The drawing under review shows one solid part. Ordinate dimensions are in mm from its lowest x, y, z. A direction names the side the tool comes from. Give positions to 0.01 mm unless a question says otherwise; leave off trailing zeros. Write each loop counter-clockwise with the first axis right and the second up, starting at its lowest first coordinate (ties: lowest second). Pieces come first, ordered by that corner, then holes. Notation, with made-up numbers: (85.5, 4.5) -> (104.5, 4.5) arc R23 cw to (104.5, 29.5) -> close; hole circle Ø4 at (-1, -13.75). An arc over 180 degrees is marked (long way). Write item = value, one per line.
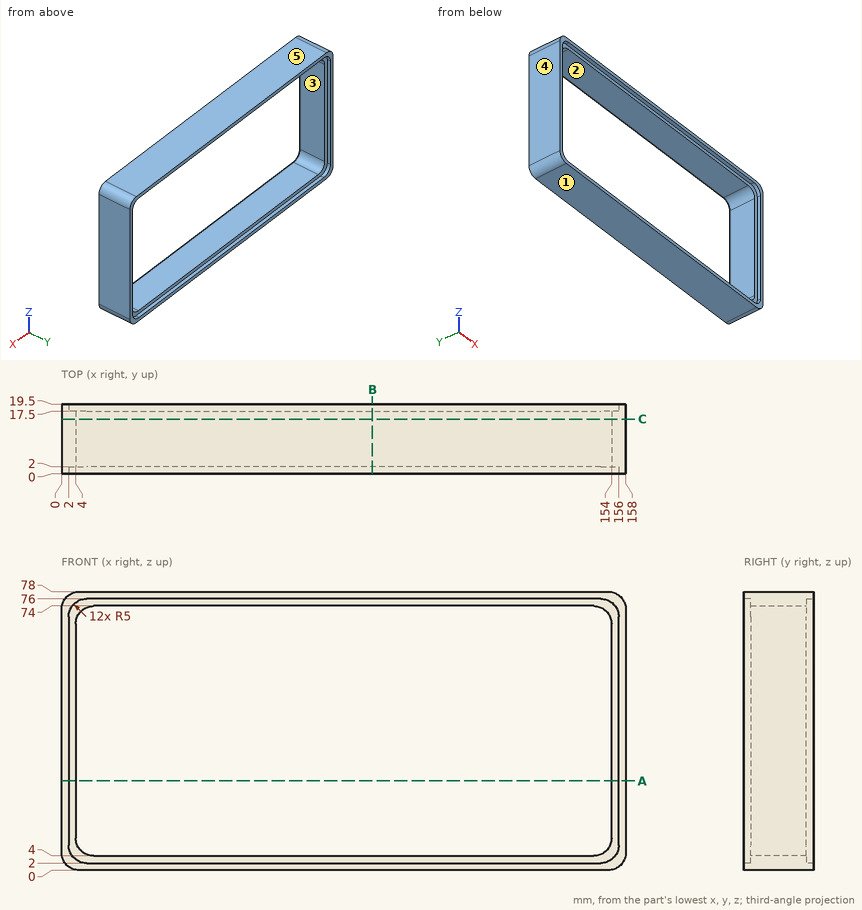
(1) Take a section at C-C (y = 15.25). Write out the cut boundary in (x, z).
Answers below:
outline = (0, 5) arc R5 ccw to (5, 0) -> (153, 0) arc R5 ccw to (158, 5) -> (158, 73) arc R5 ccw to (153, 78) -> (5, 78) arc R5 ccw to (0, 73) -> close; hole (4, 9) arc R5 ccw to (9, 4) -> (149, 4) arc R5 ccw to (154, 9) -> (154, 69) arc R5 ccw to (149, 74) -> (9, 74) arc R5 ccw to (4, 69) -> close
(2) Take a section at B-B (x = 87). Write out the cut boundary in (y, z), plus the area to 3 significant figures.
Answers below:
outline = (0, 0) -> (19.5, 0) -> (19.5, 2) -> (17.5, 2) -> (17.5, 4) -> (2, 4) -> (2, 2) -> (0, 2) -> close; (0, 76) -> (2, 76) -> (2, 74) -> (17.5, 74) -> (17.5, 76) -> (19.5, 76) -> (19.5, 78) -> (0, 78) -> close
area = 140 mm^2
(3) Take a section at A-A (z = 25). Write out the cut boundary in (x, y), plus the area to 3 significant figures.
Answers below:
outline = (0, 0) -> (2, 0) -> (2, 2) -> (4, 2) -> (4, 17.5) -> (2, 17.5) -> (2, 19.5) -> (0, 19.5) -> close; (154, 2) -> (156, 2) -> (156, 0) -> (158, 0) -> (158, 19.5) -> (156, 19.5) -> (156, 17.5) -> (154, 17.5) -> close
area = 140 mm^2
(4) For pin 1 (2 mm diameter, centred on x = 77, y = 18, fed in from -Z), flat-tipped, find the tip position at first contact; note if it passes through.
Answers below:
pin_1 = 0
(5) The part is to be moulded in two halves that separate along Z. For the marked faces 3, 4 and 5, say which applies: released by +Z, released by -Z, zero draft, split by the parting line, or undercut.
Answers below:
face_3 = undercut
face_4 = zero draft
face_5 = released by +Z
(6) Tool access review of the marked faces 1 and 2: name each direction out of +Z, -Z, +X, -X, +Y, -Y from which nothing blocks a thin tool from reaching the whole face with its end or side.
Answers below:
face_1 = -Z, +X, -X, +Y, -Y
face_2 = +Y, -Y
(7) To check wall thickness, follow probe 1 along Z at (x, y) = (125, 4); probe 2 along X at (y, z) = (8.25, 11); probe 3 along X at (y, z) = (18.5, 10.5). State the ranges of each line that lie inside material, in increasing order.
Answers below:
probe_1 = 0 to 4, 74 to 78
probe_2 = 0 to 4, 154 to 158
probe_3 = 0 to 2, 156 to 158
